Could you check a few things on this model? Use its own coordinates, in mm. Face numbers are marked on the shaded views. Coordinates: 2 decimals unless noted, no trailing zeros. Order: outer loops, then holes, each group sorted by start corner. A loop starts at its lowest first (then second) coordinate and runs counter-clockwise, first axis right, second up. Notation, with made-up numbers: (-39.5, 30.5) -> (-5.5, 30.5) arc R18 ccw to (-5.5, 40.5) -> close; hole circle Ø2 at (29, 81). An arc over 180 degrees is marked (long way). Return JSON: item names as keys, results as strings. Group by question number.
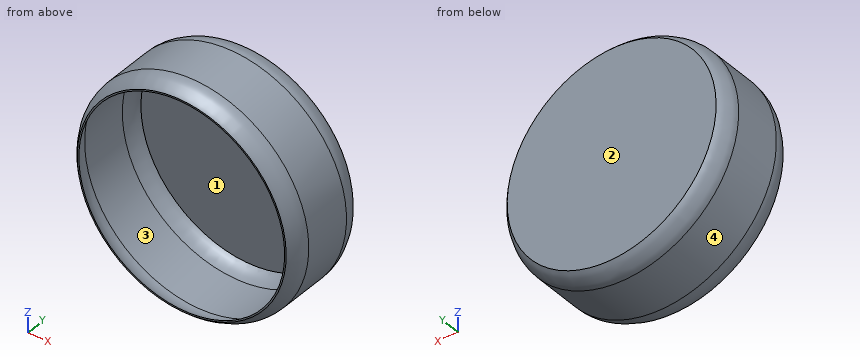
from build123d import *

# Parameters (mm, degrees)
ENL_V_START             = -0.2
ESQUISSE2_R             = 1
ENL_V_MAT_EXTRU_1_DEPTH = 0.4


# Read off the part's stored shape, not the designer's step: Coque1
with BuildPart() as part:
    # Esquisse1 → Révolution1 (revolve)
    with BuildSketch(Plane.XY, mode=Mode.PRIVATE) as r_volution1_sk:
        with BuildLine():
            Line((0, 0), (0, 34))
            Line((0, 34), (41.75, 34))
            ThreePointArc((41.75, 34), (44.151502609, 30.652951592), (45, 26.621822718))
            Line((45, 26.621822718), (45, 7.378177282))
            ThreePointArc((45, 7.378177282), (44.151502609, 3.347048408), (41.75, 0))
            Line((41.75, 0), (0, 0))
        make_face()
    revolve(r_volution1_sk.sketch.rotate(Axis((0, 34, 0), (0, 1, 0)), 90), axis=Axis((0, 34, 0), (0, 1, 0)))

    # Coque1 outline → Coque1 (revolve, cut)
    with BuildSketch(Plane.XY):
        with BuildLine():
            Line((44.6, 7.378177282), (44.6, 26.621822718))
            ThreePointArc((44.6, 26.621822718), (43.973260711, 30.033653928), (42.174876624, 33))
            Line((42.174876624, 33), (0, 33))
            Line((0, 33), (0, 0))
            Line((0, 0), (41.141864538, 0))
            ThreePointArc((41.141864538, 0), (43.692580157, 3.303984083), (44.6, 7.378177282))
        make_face()
    revolve(axis=Axis((0, 0, 0), (0, 1, 0)), mode=Mode.SUBTRACT)

    # Esquisse2 → Enlèv. mat.-Extru.1 (cut)
    with BuildSketch(Plane(origin=(0, 34, 0), x_dir=(1, 0, 0), z_dir=(0, 1, 0)).offset(ENL_V_START)):
        with Locations(Location((-31.5, 0, 0), (0, 0, 270))):
            Circle(ESQUISSE2_R)
        with Locations(Location((31.5, 0, 0), (0, 0, 90))):
            Circle(ESQUISSE2_R)
    extrude(amount=-ENL_V_MAT_EXTRU_1_DEPTH, mode=Mode.SUBTRACT)


solid = part.part
Q1. I need wall thicknesses on line 1 along X through (y, z) = (18.75, 0); line 2 along Y through (x, z) = (30, 28); line 3 along Z through (x, y) = (-28, 15). Which ranges of each line are inside material? Lowest first, please. Write a range as from..to.
Q2. We'd pull the mould along X, two halves only. Please class the marked faces 1, 2, 3 and 4: pulls with the +X half, pulls with the -X half, needs draft (parallel to the pull), parting line crosses it, or undercut.
Q3. I want a section at B-B on x = 0. Please give me the cut outline in (y, z), and give its area (3 significant figures).
Q4. I want a section at A-A on y = 15.5. Please give me the cut outline in (x, z).
Q5. I want a section at C-C on y = 31.5. Please give me the cut outline in (x, z).
Q6. I'm going to push flat-ended pins straight in: pin 1 Ø2 at (x, y) = (28.5, 14.5) entering from +Z; pin 2 Ø12 at (x, y) = (10, 26) entering from -Z; pin 3 Ø3 at (x, y) = (11.5, 3.5) entering from +Z. Where does each tip first touch, or does it pass through?
Response values:
{
 "1": {"line 1": "x = -45..-44.6, 44.6..45", "line 2": "y = 33..34", "line 3": "z = -35.23..-34.72, 34.72..35.23"},
 "2": {"face 1": "undercut", "face 2": "needs draft", "face 3": "undercut", "face 4": "parting line crosses it"},
 "3": {"outline": "(0, -41.75) arc R10 ccw to (7.38, -45) -> (26.62, -45) arc R10 ccw to (34, -41.75) -> (34, 41.75) arc R10 ccw to (26.62, 45) -> (7.38, 45) arc R10 ccw to (0, 41.75) -> (0, 41.14) arc R9.6 cw to (7.38, 44.6) -> (26.62, 44.6) arc R9.6 cw to (33, 42.17) -> (33, -42.17) arc R9.6 cw to (26.62, -44.6) -> (7.38, -44.6) arc R9.6 cw to (0, -41.14) -> close", "area": "112 mm²"},
 "4": {"outline": "circle Ø90 at (0, 0); hole circle Ø89.2 at (0, 0)"},
 "5": {"outline": "circle Ø87.46 at (0, 0); hole circle Ø86.54 at (0, 0)"},
 "6": {"pin 1": "stops at z = 35.62", "pin 2": "stops at z = -44.82", "pin 3": "stops at z = 43.36"}
}
